Geometry check sheet. Reference: the model listing, model coordinates, mm. A direction names the side the tool comes from. Coordinates: 2 decimals unless noted, no trailing zeros. Loops run counter-clockwise (first coordinate to the right, second up) from the corner with the lowest first, then second, coordinate; pieces in that order, holes last. Notation, with made-up numbers: M 45,-17 L 97,-17 A11 cw 97,-1 Z; hole C 26,68 d11. An arc over 180 degrees is marked long. Use CSV: the item, a comma, the result in double quotes.
```python
from build123d import *

# Parameters (mm, degrees)
SKETCH_1_W          = 50
SKETCH_1_H          = 50
SKETCH_1_R          = 10
SKETCH_1_W_2        = 82
SKETCH_1_H_2        = 15
EXTRUDE_1_DEPTH     = 19
FILLET_1_R          = 21
FILLET_3_R          = 21
SKETCH_2_R          = 4.5
CUT_EXTRUDE_1_DEPTH = 19


with BuildPart() as part:
    # 草图1 → 凸台-拉伸1 (new body)
    with BuildSketch(Plane.XY):
        with Locations((0, 32.5)):
            Rectangle(SKETCH_1_W, SKETCH_1_H)
        with Locations((0, 32.5)):
            Circle(SKETCH_1_R, mode=Mode.SUBTRACT)
        Rectangle(SKETCH_1_W_2, SKETCH_1_H_2)
    extrude(amount=EXTRUDE_1_DEPTH)

    # 圆角1
    fillet_1_edges = [part.edges().sort_by_distance(p)[0] for p in [
        (-25, 57.5, 9.5),
    ]]
    fillet(fillet_1_edges, radius=FILLET_1_R)

    # 圆角3
    fillet_3_edges = [part.edges().sort_by_distance(p)[0] for p in [
        (25, 57.5, 9.5),
    ]]
    fillet(fillet_3_edges, radius=FILLET_3_R)

    # 草图2 → 切除-拉伸1 (cut)
    with BuildSketch(Plane.XZ.offset(7.5)):
        with Locations((-33, 9.5)):
            Circle(SKETCH_2_R)
        with Locations((33, 9.5)):
            Circle(SKETCH_2_R)
    extrude(amount=-CUT_EXTRUDE_1_DEPTH, mode=Mode.SUBTRACT)


solid = part.part
```
1. Release check for a two-part mould opening along Y. For faces 1 (the cylindrical face through (-19.012, 51.185, 9.633)), 2 (the cylindrical face through (-2.17, 22.74, 9.37)), 3 (the cylindrical face through (-28.708, -0.105, 10.852)) record: +Y half, -Y half, draft (parallel to the pull), parting line (faces both ways), or undercut.
The answers:
face 1,"+Y half"
face 2,"undercut"
face 3,"draft"
2. Section check D-D, the plane y = 4. Record the cut outline in (x, z), plus the area to 3 significant figures.
The answers:
outline,"M -41,0 L 41,0 L 41,19 L -41,19 Z; hole C -33,9.5 d9; hole C 33,9.5 d9"
area,"1,430 mm^2"
3. Section check C-C, the plane x = 0. Record the cut outline in (y, z).
The answers:
outline,"M -7.5,0 L 22.5,0 L 22.5,19 L -7.5,19 Z; M 42.5,0 L 57.5,0 L 57.5,19 L 42.5,19 Z"
4. Set-up check for faces 4 (the flat face through (-35, 7.5, 5)), 5 (the flat face through (0, 57.5, 9)), 6 (the flat face through (25, 22, 9)): record each of +Z, -Z, +X, -X, +Y, -Y from which the full face is reachable in a straight line by a thin tool's end or side.
The answers:
face 4,"+Z, -Z, -X, +Y"
face 5,"+Z, -Z, +X, -X, +Y"
face 6,"+Z, -Z, +X, +Y"
5. Section check A-A, the plane z = 9.5. Record the cut outline in (x, y), plus the area to 3 significant figures.
The answers:
outline,"M -41,-7.5 L -37.5,-7.5 L -37.5,7.5 L -41,7.5 Z; M -28.5,-7.5 L 28.5,-7.5 L 28.5,7.5 L 25,7.5 L 25,36.5 A21 ccw 4,57.5 L -4,57.5 A21 ccw -25,36.5 L -25,7.5 L -28.5,7.5 Z; M 37.5,-7.5 L 41,-7.5 L 41,7.5 L 37.5,7.5 Z; hole C 0,32.5 d20"
area,"2,960 mm^2"
6. Thickness scan on line 1 (Z direction, x = -33, y = 0); line 2 (Y direction, x = 0.5, z = 8); line 3 (X direction, y = 0, z = 5.75). Record the ranges inside material, lowest first. Write a range as [from, to].
The answers:
line 1,"[0, 5], [14, 19]"
line 2,"[-7.5, 22.51], [42.49, 57.5]"
line 3,"[-41, -35.49], [-30.51, 30.51], [35.49, 41]"
7. Gauge pin test, flat ends, axial feed: P1, Ø8, axis at x = 33.5, z = 11, coming from the +Y side; P2, Ø1.5, axis at x = -10.5, z = 12, coming from the +Y side; P3, Ø5.5, axis at y = 27.5, z = 8.5, coming from the +X side. Record the tip position at first contact, or that the pin passes through.
The answers:
P1,"y = 7.5"
P2,"y = 56.7"
P3,"x = 25"
8. Section check B-B, the plane y = 32.5. Record the cut outline in (x, z).
The answers:
outline,"M -25,0 L -10,0 L -10,19 L -25,19 Z; M 10,0 L 25,0 L 25,19 L 10,19 Z"
